Part model, mm, in its own coordinate system. A direction names the side the tool comes from. Coordinates: 2 decimals unless noted, no trailing zeros. Write each loop counter-clockwise with the first axis right and the second up, starting at its lowest first coordinate (ties: lowest second). Pieces come first, ordered by that corner, then holes. Notation, with made-up numbers: (-40, -37) -> (7, -37) arc R9 cw to (7, -23) -> close; hole circle Ø2 at (65, 30.5). An arc over 180 degrees is marked (long way). Write item = value, one per line. Start each with the question number.
Q1. Band-saw the part on C-C, the plane x = 36.5. List the corners of the cut face in (y, z), plus the area to 3 significant figures.
Q2. Pin check, flat tips, straight feed: P1, Ø1.5, axis at x = 29, y = 2, coming from the +Z side; P2, Ø1.5, axis at x = 40, z = 4, coming from the -Y side; P3, Ø2, axis at x = 45, y = 1, coming from the -Z side; P4, Ø2.5, axis at y = 3, z = 84, coming from the -X side. Stop position of each tip, or through.
Q3. Tool access for faces 4 (the flat face through (14.27, 2, 80)), 5 (the flat face through (-20, 2, 92.489)), 6 (the flat face through (-105.73, 2, -45)): list every direction of +Z, -Z, +X, -X, +Y, -Y with a clear straight run to the whole face (end or side of a thin tool).
Q4. Probe line 1 (X direction, y = 1.85, z = -47); line 2 (Z direction, x = 52, y = 3.8). List the from-to ranges inside material, lowest first.
Q5. Band-saw the part on B-B, the plane y = 2.4. List the corners of the cut face in (x, z), plus the area to 3 significant figures.
Q6. Band-saw the part on A-A, the plane z = -41. List the corners of the cut face in (x, y), plus the area to 3 significant figures.
Q7. Pull direction X, two halves, no side cores. Call faces 1 (the flat face through (-105.73, 2, 80)), 2 (the flat face through (-19, 0, 16)), 3 (the cylindrical face through (101.26, 2.46, -54.66)): released by +X, released by -X, zero draft, split by the parting line, or undercut.
from build123d import *

# Parameters (mm, degrees)
BOSS_EXTRUDE1_DEPTH = 5


with BuildPart() as part:
    # Sketch1 → Boss-Extrude1 (new body)
    with BuildSketch(Plane(origin=(0, 0, 0), x_dir=(1, 0, 0), z_dir=(0, 1, 0))):
        with BuildLine():
            Line((64.270386266, 57.510729614), (94.270386266, 57.510729614))
            ThreePointArc((94.270386266, 57.510729614), (101.341454078, 54.581797426), (104.270386266, 47.510729614))
            Line((104.270386266, 47.510729614), (104.270386266, -82.489270386))
            ThreePointArc((104.270386266, -82.489270386), (101.341454078, -89.560338198), (94.270386266, -92.489270386))
            Line((94.270386266, -92.489270386), (64.270386266, -92.489270386))
            Line((64.270386266, -92.489270386), (64.270386266, -67.489270386))
            Line((64.270386266, -67.489270386), (14.270386266, -67.489270386))
            Line((14.270386266, -67.489270386), (14.270386266, -92.489270386))
            Line((14.270386266, -92.489270386), (-55.729613734, -92.489270386))
            Line((-55.729613734, -92.489270386), (-55.729613734, -67.489270386))
            Line((-55.729613734, -67.489270386), (-105.729613734, -67.489270386))
            Line((-105.729613734, -67.489270386), (-105.729613734, -92.489270386))
            Line((-105.729613734, -92.489270386), (-135.729613734, -92.489270386))
            ThreePointArc((-135.729613734, -92.489270386), (-142.800681546, -89.560338198), (-145.729613734, -82.489270386))
            Line((-145.729613734, -82.489270386), (-145.729613734, 47.510729614))
            ThreePointArc((-145.729613734, 47.510729614), (-142.800681546, 54.581797426), (-135.729613734, 57.510729614))
            Line((-135.729613734, 57.510729614), (-105.729613734, 57.510729614))
            Line((-105.729613734, 57.510729614), (-105.729613734, 32.510729614))
            Line((-105.729613734, 32.510729614), (-55.729613734, 32.510729614))
            Line((-55.729613734, 32.510729614), (-55.729613734, 57.510729614))
            Line((-55.729613734, 57.510729614), (14.270386266, 57.510729614))
            Line((14.270386266, 57.510729614), (14.270386266, 32.510729614))
            Line((14.270386266, 32.510729614), (64.270386266, 32.510729614))
            Line((64.270386266, 32.510729614), (64.270386266, 57.510729614))
        make_face()
    extrude(amount=BOSS_EXTRUDE1_DEPTH)


solid = part.part
Ans:
q1.outline = (0, -32.51) -> (5, -32.51) -> (5, 67.49) -> (0, 67.49) -> close
q1.area = 500 mm2
q2.P1 = 67.49
q2.P2 = 0
q2.P3 = -32.51
q2.P4 = -145.73
q3.face_4 = +Z, +Y, -Y
q3.face_5 = +Z, +X, -X, +Y, -Y
q3.face_6 = -Z, +Y, -Y
q4.line_1 = -145.73 to -105.73, -55.73 to 14.27, 64.27 to 104.27
q4.line_2 = -32.51 to 67.49
q5.outline = (-145.73, -47.51) arc R10 ccw to (-135.73, -57.51) -> (-105.73, -57.51) -> (-105.73, -32.51) -> (-55.73, -32.51) -> (-55.73, -57.51) -> (14.27, -57.51) -> (14.27, -32.51) -> (64.27, -32.51) -> (64.27, -57.51) -> (94.27, -57.51) arc R10 ccw to (104.27, -47.51) -> (104.27, 82.49) arc R10 ccw to (94.27, 92.49) -> (64.27, 92.49) -> (64.27, 67.49) -> (14.27, 67.49) -> (14.27, 92.49) -> (-55.73, 92.49) -> (-55.73, 67.49) -> (-105.73, 67.49) -> (-105.73, 92.49) -> (-135.73, 92.49) arc R10 ccw to (-145.73, 82.49) -> close
q5.area = 32,400 mm2
q6.outline = (-145.73, 0) -> (-105.73, 0) -> (-105.73, 5) -> (-145.73, 5) -> close; (-55.73, 0) -> (14.27, 0) -> (14.27, 5) -> (-55.73, 5) -> close; (64.27, 0) -> (104.27, 0) -> (104.27, 5) -> (64.27, 5) -> close
q6.area = 750 mm2
q7.face_1 = undercut
q7.face_2 = zero draft
q7.face_3 = released by +X
